Check sheet for the modelled part. Datum: model origin and axes. Units: mm. Face numbers are marked on the shaded views. Round coordinates to 2 decimals unless told otherwise and drop trailing zeros. Order: outer loops, then holes, each group sorted by start corner. A loop starts at its lowest first (then second) coordinate and runs counter-clockwise, first axis right, second up.
(1) Sectioned sample at C-C, the plane y = 8.25. Enter the section's corners in (x, z).
(2) Depth check by flat-ended pin: pin 1 (0.7 mm diameter, centred on y = -5, z = 2, fed in from +X); pin 2 (0.7 mm diameter, centred on y = 8, z = 1, fed in from -X); pin 3 (1.2 mm diameter, centred on x = 30.15, y = 0, fed in from +Z); pin 4 (1.2 mm diameter, centred on x = 25.5, z = 2, fed in from +Y). Enter the tip coordinate at first touch or a pass-through.
(3) Sectioned sample at D-D, the plane y = 3.5. Enter the section's corners in (x, z).
(4) Sectioned sample at B-B, the plane z = 1.35. Enter the section's corners in (x, y), and give its area (3 significant figures).
(5) Thickness scan on probe 1 along Y at (x, z) = (30, 1.15); probe 2 along X at (y, z) = (7.5, 0.4); probe 3 along Y at (x, z) = (30.5, 1.05). Record the ranges inside material, lowest first.
(6) Sectioned sample at A-A, the plane y = 0. Enter the section's corners in (x, z), and give its area (3 significant figures).
(7) Mould release check, pull along Z, two halves, no side actions. Record for the marked faces 1 and 2: released by +Z, released by -Z, zero draft, split by the parting line, or undercut.
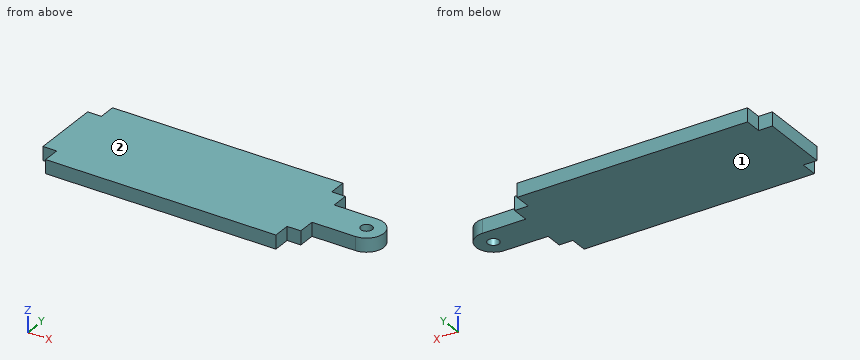
```python
from build123d import *

# Parameters (mm, degrees)
SKETCH1_R           = 1
BOSS_EXTRUDE1_DEPTH = 2.4


with BuildPart() as part:
    # Sketch1 → Boss-Extrude1 (new body)
    with BuildSketch(Plane.XY):
        with BuildLine():
            Line((22.55, -3), (30.15, -3))
            ThreePointArc((30.15, -3), (33.15, 0), (30.15, 3))
            Line((30.15, 3), (22.55, 3))
            Line((22.55, 3), (22.55, 6))
            Line((22.55, 6), (20.15, 6))
            Line((20.15, 6), (20.15, 9))
            Line((20.15, 9), (-20.15, 9))
            Line((-20.15, 9), (-20.15, 6))
            Line((-20.15, 6), (-22.55, 6))
            Line((-22.55, 6), (-22.55, -6))
            Line((-22.55, -6), (-20.15, -6))
            Line((-20.15, -6), (-20.15, -9))
            Line((-20.15, -9), (20.15, -9))
            Line((20.15, -9), (20.15, -6))
            Line((20.15, -6), (22.55, -6))
            Line((22.55, -6), (22.55, -3))
        make_face()
        with Locations((30.15, 0)):
            Circle(SKETCH1_R, mode=Mode.SUBTRACT)
    extrude(amount=BOSS_EXTRUDE1_DEPTH)


solid = part.part
```
Derived:
1. outline: (-20.15, 0) - (20.15, 0) - (20.15, 2.4) - (-20.15, 2.4) - close
2. pin 1: stops at x = 22.55
2. pin 2: stops at x = -20.15
2. pin 3: passes through
2. pin 4: stops at y = 3
3. outline: (-22.55, 0) - (22.55, 0) - (22.55, 2.4) - (-22.55, 2.4) - close
4. outline: (-22.55, -6) - (-20.15, -6) - (-20.15, -9) - (20.15, -9) - (20.15, -6) - (22.55, -6) - (22.55, -3) - (30.15, -3) arc R3 ccw to (30.15, 3) - (22.55, 3) - (22.55, 6) - (20.15, 6) - (20.15, 9) - (-20.15, 9) - (-20.15, 6) - (-22.55, 6) - close; hole circle Ø2 at (30.15, 0)
4. area: 840 mm2
5. probe 1: y = -3 to -0.99, 0.99 to 3
5. probe 2: x = -20.15 to 20.15
5. probe 3: y = -2.98 to -0.94, 0.94 to 2.98
6. outline: (-22.55, 0) - (29.15, 0) - (29.15, 2.4) - (-22.55, 2.4) - close; (31.15, 0) - (33.15, 0) - (33.15, 2.4) - (31.15, 2.4) - close
6. area: 129 mm2
7. face 1: released by -Z
7. face 2: released by +Z
